Read the model definition and answer for the solid it produces. Units are mm, in the model's axes. Face numbers are marked on the shaded views. Coordinates: 2 decimals unless noted, no trailing zeros. Write each loop counter-clockwise with the first axis right and the second up, starting at its lowest first coordinate (ties: lowest second). Pieces come first, ordered by that corner, then holes.
(1) The mould has two halves that part along Y. Classify the marked faces 1 and 2: +Y half, -Y half, draft (parallel to the pull), parting line (faces both ways), or undercut.
(2) Find the intervals of material crossed by probe 1 along Y at (x, z) = (0, 0.5) (3 decimals); probe 2 along X at (y, z) = (2, 0.65); probe 3 along X at (y, z) = (1, -0.5) (3 decimals), in increasing order.
(3) Section C-C on y = 6 is taken. Write down the section's boundary in (x, z) (3 decimals), then the cut area to 3 significant figures.
(4) Section D-D on x = -9 is taken. Write down the section's boundary in (y, z) (3 decimals), then the cut area to 3 significant figures.
(5) Given pin 1 (6.5 mm diameter, centred on x = 0, y = 0, fed in from +Z); pin 2 (6 mm diameter, centred on x = 5, y = 4, fed in from -Z); pin 3 (0.9 mm diameter, centred on x = 1.5, z = -1, fed in from -Y); pin 4 (0.9 mm diameter, centred on y = 5, z = -1, fed in from +X), each flat-ended and moving along its own axis, determine where each tip first touches the part or whether it passes through.
(6) Section A-A on y = 0 is taken. Write down the section's boundary in (x, z) (3 decimals), then the cut area to 3 significant figures.
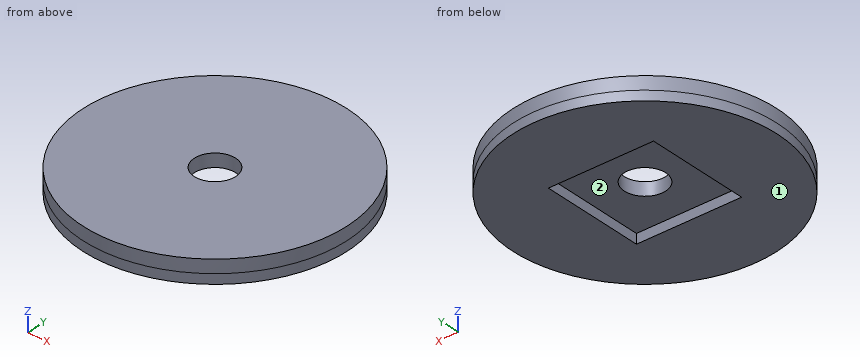
Autodesk Inventor part; units mm, degrees
ref_plane "Work Plane1" through (7, -9.9, -1.8716) normal (0, 0, -1) x (0, 1, 0)
ref_plane "YZ Plane" through (0, 0, 0) normal (1, 0, 0) x (0, 1, 0)
ref_plane "XZ Plane" through (0, 0, 0) normal (0, 1, 0) x (-1, 0, 0)
sketch "Sketch1" plane through (0, 0, 0) normal (0, 0, 1) x (1, 0, 0)
  line L0 (-25.4, 25.4) -> (25.4, 25.4)
  line L1 (25.4, 25.4) -> (25.4, -25.4)
  line L2 (25.4, -25.4) -> (-25.4, -25.4)
  line L3 (-25.4, -25.4) -> (-25.4, 25.4)
  line L4 (-25.4, 25.4) -> (25.4, -25.4) construction
  line L5 (25.4, 25.4) -> (-25.4, -25.4) construction
  circle A0 centre (0, 0) radius 25.4
  dimension "d0" = 50.8
  dimension "d1" = 50.8
extrude "Extrusion1" add sketch "Sketch1" along normal blind 2.54 contours A0
sketch "Sketch2" plane through (0, 0, 2.54) normal (0, 0, 1) x (1, 0, 0)
  circle A0 centre (0, 0) radius 3.975
extrude "Extrusion2" cut sketch "Sketch2" against normal blind 2.54
sketch "Sketch3" plane through (0, 0, 0) normal (0, 0, -1) x (-1, 0, 0)
  line L0 (-10, 10) -> (-10, -10)
  line L1 (10, 9.9) -> (10, -9.9)
  line L2 (7, -10) -> (-7, -10)
  line L3 (-7, 10) -> (7, 10)
  line L4 (-10.125, -10.125) -> (10.125, -10.125)
  line L5 (10.125, -10.125) -> (10.125, 10.125)
  line L6 (10.125, 10.125) -> (-10.125, 10.125)
  line L7 (-10.125, 10.125) -> (-10.125, -10.125)
  line L8 (-10.125, -10.125) -> (10.125, 10.125) construction
  line L9 (10.125, -10.125) -> (-10.125, 10.125) construction
  circle A0 centre (0, 0) radius 3.975
  circle A1 centre (0, 0) radius 3.975
  circle A2 centre (0, 0) radius 25.4
  dimension "d6" = 20.25
  dimension "d7" = 20.25
ref_plane "Work Plane1" through (7, -9.9, -1.8716) normal (0, 0, -1) x (0, 1, 0)
extrude "Extrusion3" add sketch "Sketch3" along normal up to surface (1.8716 mm away) contours A2
properties part number "Base"
Response:
1. face 1: draft
1. face 2: undercut
2. probe 1: y = -25.4 to -3.975, 3.975 to 25.4
2. probe 2: x = -25.32 to -3.44, 3.44 to 25.32
2. probe 3: x = -25.38 to -10.125, 10.125 to 25.38
3. outline: (-24.681, -1.872) - (-10.125, -1.872) - (-10.125, 0) - (10.125, 0) - (10.125, -1.872) - (24.681, -1.872) - (24.681, 2.54) - (-24.681, 2.54) - close
3. area: 180 mm2
4. outline: (-23.752, -1.872) - (-10.125, -1.872) - (-10.125, 0) - (10.125, 0) - (10.125, -1.872) - (23.752, -1.872) - (23.752, 2.54) - (-23.752, 2.54) - close
4. area: 172 mm2
5. pin 1: passes through
5. pin 2: stops at z = 0
5. pin 3: stops at y = -25.38
5. pin 4: stops at x = 24.99
6. outline: (-25.4, -1.872) - (-10.125, -1.872) - (-10.125, 0) - (-3.975, 0) - (-3.975, 2.54) - (-25.4, 2.54) - close; (3.975, 0) - (10.125, 0) - (10.125, -1.872) - (25.4, -1.872) - (25.4, 2.54) - (3.975, 2.54) - close
6. area: 166 mm2
